```python
from build123d import *

# Parameters (mm, degrees)
CYLINDER072_R     = 1.5
CYLINDER072_DEPTH = 4
CYLINDER071_R     = 1.5
CYLINDER071_DEPTH = 4
CYLINDER073_R     = 1.5
CYLINDER073_DEPTH = 4
CYLINDER070_R     = 1.5
CYLINDER070_DEPTH = 4
EXTRUDE004_DEPTH  = 10
FILLET007_R       = 0.5
BOX017_W          = 3
BOX017_H          = 20
BOX017_DEPTH      = 5
FILLET009_R       = 2
BOX016_W          = 30
BOX016_H          = 73
BOX016_DEPTH      = 4
FILLET008_R       = 2


with BuildPart() as payload_plate_screw009:
    # Cylinder072 → Cylinder072 (new body)
    with BuildSketch(Plane(origin=(-10, 25, 152.7), x_dir=(1, 0, 0), z_dir=(0, 0, 1))):
        Circle(CYLINDER072_R)
    extrude(amount=CYLINDER072_DEPTH)


with BuildPart() as payload_plate_screw008:
    # Cylinder071 → Cylinder071 (new body)
    with BuildSketch(Plane(origin=(-10, -33, 152.7), x_dir=(1, 0, 0), z_dir=(0, 0, 1))):
        Circle(CYLINDER071_R)
    extrude(amount=CYLINDER071_DEPTH)


with BuildPart() as payload_plate_screw010:
    # Cylinder073 → Cylinder073 (new body)
    with BuildSketch(Plane(origin=(10, 25, 152.7), x_dir=(1, 0, 0), z_dir=(0, 0, 1))):
        Circle(CYLINDER073_R)
    extrude(amount=CYLINDER073_DEPTH)


with BuildPart() as payload_plate_screw_holes001:
    # Cylinder070 → Cylinder070 (new body)
    with BuildSketch(Plane(origin=(10, -33, 152.7), x_dir=(1, 0, 0), z_dir=(0, 0, 1))):
        Circle(CYLINDER070_R)
    extrude(amount=CYLINDER070_DEPTH)

    # Compound009: union payload-plate-screw009, payload-plate-screw008, payload-plate-screw010
    add(payload_plate_screw009.part)
    add(payload_plate_screw008.part)
    add(payload_plate_screw010.part)


with BuildPart() as webcam_cradle:
    # Sketch → Extrude004 (new body, symmetric)
    with BuildSketch(Plane.XZ):
        with BuildLine():
            Line((-9.5, 0), (9.5, 0))
            Line((9.5, 0), (9.5, 6.5))
            ThreePointArc((-9.5, 1), (0.468514, 2.131496), (9.5, 6.5))
            Line((-9.5, 0), (-9.5, 1))
        make_face()
    extrude(amount=EXTRUDE004_DEPTH, both=True)

    # Fillet007
    fillet007_edges = [webcam_cradle.edges().sort_by_distance(p)[0] for p in [
        (9.5, 0, 6.5),
    ]]
    fillet(fillet007_edges, radius=FILLET007_R)


with BuildPart() as webcam_cradle_1:
    # Fillet007 placement: moved
    add(webcam_cradle.part.moved(Location((0, 0, 156.7))))


with BuildPart() as from_stop:
    # Box017 → Box017 (new body)
    with BuildSketch(Plane(origin=(-12.5, -10, 156.7), x_dir=(1, 0, 0), z_dir=(0, 0, 1))):
        with Locations((1.5, 10)):
            Rectangle(BOX017_W, BOX017_H)
    extrude(amount=BOX017_DEPTH)

    # Fillet009
    fillet009_edges = [from_stop.edges().sort_by_distance(p)[0] for p in [
        (-12.5, 0, 161.7),
    ]]
    fillet(fillet009_edges, radius=FILLET009_R)


with BuildPart() as payload_plate_webcam:
    # Box016 → Box016 (new body)
    with BuildSketch(Plane(origin=(-15, -40.5, 152.7), x_dir=(1, 0, 0), z_dir=(0, 0, 1))):
        with Locations((15, 36.5)):
            Rectangle(BOX016_W, BOX016_H)
    extrude(amount=BOX016_DEPTH)

    # Fusion030: union webcam-cradle, from-stop
    add(webcam_cradle_1.part)
    add(from_stop.part)

    # Fillet008
    fillet008_edges = [payload_plate_webcam.edges().sort_by_distance(p)[0] for p in [
        (0, -40.5, 156.7),
        (0, 32.5, 156.7),
    ]]
    fillet(fillet008_edges, radius=FILLET008_R)

    # Cut054: cut payload-plate-screw-holes001
    add(payload_plate_screw_holes001.part, mode=Mode.SUBTRACT)


solid = payload_plate_webcam.part
```
Verification items for the finished model (mm, model axes). A direction names the side the tool comes from. Round coordinates to 2 decimals unless told otherwise and drop trailing zeros. Write each loop counter-clockwise with the first axis right and the second up, starting at its lowest first coordinate (ties: lowest second). Pieces come first, ordered by that corner, then holes.
1. Section check B-B on z = 158.5. Enter the section's corners in (x, y), plus the area to 3 significant figures.
2. Section check C-C on y = -6. Enter the section's corners in (x, z), plus the area to 3 significant figures.
3. Access from +Z, -Z, +X, -X, +Y, -Y to the whole of each face (thin tool, end or side, straight path). Record for faces 1 (the cylindrical face through (-0.116, -0.14, 158.669)), 2 (the flat face through (9.5, 0, 159)), 3 (the flat face through (1, -10, 158)), 4 (the flat face through (1, 10, 158)).
4. Scan lines: L1, parallel to Y at x = 10, z = 153.8; L2, parallel to Y at x = 9.25, z = 153.75; L3, parallel to Y at x = -7.5, z = 156.75. Record each from-to range of solid material in increasing order.
5. Section check A-A on y = 25. Enter the section's corners in (x, z), plus the area to 3 significant figures.
6. Section check D-D on x = 5.5. Enter the section's corners in (y, z), plus the area to 3 significant figures.
7. Draft check along X on faces 5 (the cylindrical face through (8.8, -33.9, 154.7)), 6 (the flat face through (-9.5, 0, 160)), 7 (the cylindrical face through (0.21, 31.9, 156.13)), 8 (the flat face through (-12.5, 0, 158)). Enter one of: +X half, -X half, draft (parallel to the pull), parting line (faces both ways), or undercut.
8. Gauge pin test, flat ends, axial feed: P1, Ø5, axis at x = -10, y = 25, coming from the +Z side; P2, Ø5, axis at x = 2, z = 161, coming from the +Y side; P3, Ø1.2, axis at y = -3.5, z = 159.5, coming from the +X side; P4, Ø2.5, axis at x = 10, y = -33, coming from the +Z side (3 decimals). Record the tip position at first contact, or that the pin passes through.
Answer:
1. outline: (-12.5, -10) - (-9.5, -10) - (-9.5, 10) - (-12.5, 10) - close; (-0.78, -10) - (9.5, -10) - (9.5, 10) - (-0.78, 10) - close
1. area: 266 mm2
2. outline: (-15, 152.7) - (15, 152.7) - (15, 156.7) - (9.5, 156.7) - (9.5, 162.25) arc R0.5 ccw to (8.72, 162.66) arc R29.87 cw to (-9.5, 157.7) - (-9.5, 161.7) - (-10.5, 161.7) arc R2 ccw to (-12.5, 159.7) - (-12.5, 156.7) - (-15, 156.7) - close
2. area: 183 mm2
3. face 1: +Z, +Y, -Y
3. face 2: +Z, +X, +Y, -Y
3. face 3: +Z, +X, -X, -Y
3. face 4: +Z, +X, -X, +Y
4. L1: y = -40.5 to -34.5, -31.5 to 23.5, 26.5 to 32.5
4. L2: y = -40.5 to -34.3, -31.7 to 23.7, 26.3 to 32.5
4. L3: y = -10 to 10
5. outline: (-15, 152.7) - (-11.5, 152.7) - (-11.5, 156.7) - (-15, 156.7) - close; (-8.5, 152.7) - (8.5, 152.7) - (8.5, 156.7) - (-8.5, 156.7) - close; (11.5, 152.7) - (15, 152.7) - (15, 156.7) - (11.5, 156.7) - close
5. area: 96.0 mm2
6. outline: (-40.5, 152.7) - (32.5, 152.7) - (32.5, 154.7) arc R2 ccw to (30.5, 156.7) - (10, 156.7) - (10, 160.8) - (-10, 160.8) - (-10, 156.7) - (-38.5, 156.7) arc R2 ccw to (-40.5, 154.7) - close
6. area: 372 mm2
7. face 5: undercut
7. face 6: undercut
7. face 7: draft
7. face 8: -X half
8. P1: stops at z = 156.7
8. P2: stops at y = 10
8. P3: stops at x = 9.5
8. P4: passes through
